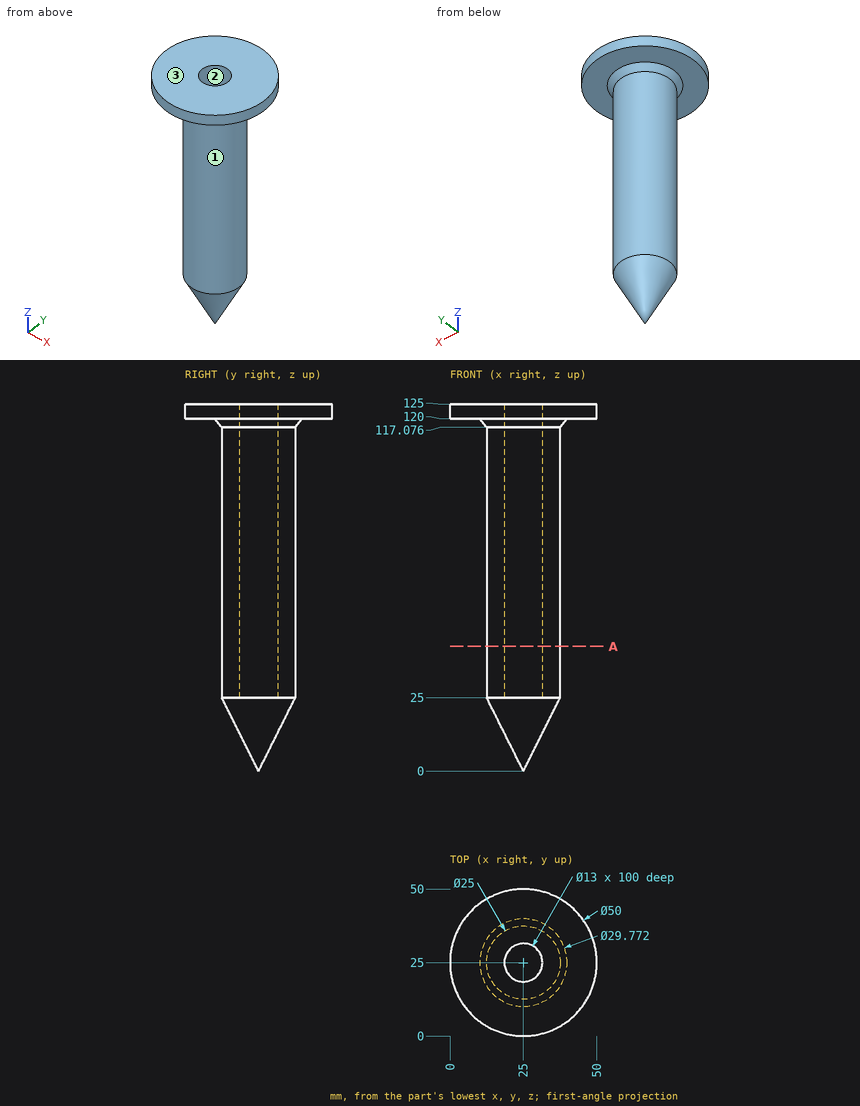
The drawing under review shows one solid part. Ordinate dimensions are in mm from its lowest x, y, z. Coordinates: 2 decimals unless noted, no trailing zeros. Order: outer loops, then holes, each group sorted by start corner. A loop starts at its lowest first (then second) coordinate and runs counter-clockwise, first axis right, second up. Notation, with made-up numbers: (55.25, 27.5) -> (80.25, 27.5) arc R12 cw to (80.25, 31.5) -> close; hole circle Ø7 at (-10.75, 12.25). An arc over 180 degrees is marked (long way). Answer as CSV lines item,"result".
Q1. Clearance check with flat-ended pins moving along their axes: pin 1 Ø10.5 at (x, y) = (25, 25) entering from +Z; pin 2 Ø15 at (x, y) = (24, 36.5) entering from -Z (1 decimal); pin 3 Ø6 at (x, z) = (25.5, 77.5) entering from +Y; pin 4 Ø5 at (x, z) = (41.5, 65.5) entering from +Y. State where each tip first meets the part, or that it passes through.
Model answer:
pin 1,"stops at z = 25"
pin 2,"stops at z = 8.1"
pin 3,"stops at y = 37.5"
pin 4,"passes through"
Q2. Wall thickness on line 1 along Y through (x, z) = (25, 105); line 2 along Z through (x, y) = (6, 35); line 3 along X through (y, z) = (30.5, 87) (1 decimal): over which ranges is each line inside the solid? List them lowest first. Write a range as [from, to].
Model answer:
line 1,"y = [12.5, 18.5], [31.5, 37.5]"
line 2,"z = [120, 125]"
line 3,"x = [13.8, 21.5], [28.5, 36.2]"
Q3. Draft analysis for pull direction X (two halves, no side actions). For the marked faces 1, 2 and 3, state which applies: released by +X, released by -X, zero draft, split by the parting line, or undercut.
Model answer:
face 1,"split by the parting line"
face 2,"undercut"
face 3,"zero draft"
Q4. We need section A-A (z = 42.5). State the section outline as (x, y) points.
Model answer:
outline,"circle Ø25 at (25, 25); hole circle Ø13 at (25, 25)"
